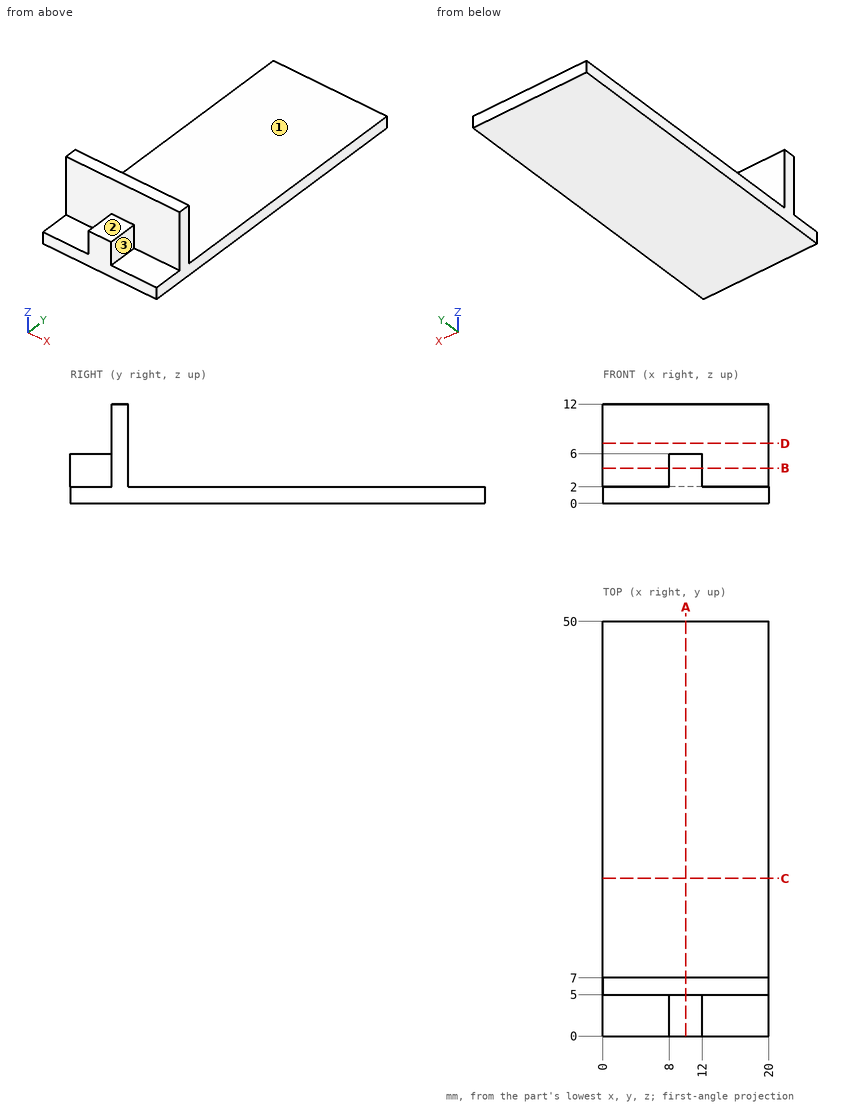
Geometry: see drawing. Coordinates: mm, zero at the bounding-box minimum. A direction names the side the tool comes from. Round coordinates to 2 decimals unless told otherwise and drop trailing zeros. Order: outer loops, then holes, each group sorted by start corner. A loop starts at its lowest first (then second) coordinate and runs counter-clockwise, first axis right, second up. Notation, with made-up numbers: (84, 3) -> (127, 3) arc R18 ccw to (127, 28) -> close; hole circle Ø7 at (86.5, -25.5). An arc over 180 degrees is marked (long way). Answer as CSV lines item,"result".
Item 1: Line query: L1, parallel to Z at x = 1.75, y = 20; L2, parallel to Y at x = 17.5, z = 11. Output: solid intervals per line, ascending.
A:
L1,"0 to 2"
L2,"5 to 7"
Item 2: Section B-B, the plane z = 4.25. Return loops of the section in (x, y), plus the area to 3 significant figures.
A:
outline,"(0, 5) -> (8, 5) -> (8, 0) -> (12, 0) -> (12, 5) -> (20, 5) -> (20, 7) -> (0, 7) -> close"
area,"60.0 mm²"
Item 3: Section A-A, the plane x = 10. Return loops of the section in (y, z).
A:
outline,"(0, 0) -> (50, 0) -> (50, 2) -> (7, 2) -> (7, 12) -> (5, 12) -> (5, 6) -> (0, 6) -> close"
Item 4: Pin query (flat end, axial travel): pin 1 Ø1.5 at (x, y) = (9.5, 13.5) entering from -Z; pin 2 Ø2 at (x, y) = (11, 1.5) entering from +Z; pin 3 Ø6 at (x, y) = (13.5, 24) entering from +Z. Return the tip coordinate at first contact, or that it passes through.
A:
pin 1,"z = 0"
pin 2,"z = 6"
pin 3,"z = 2"
Item 5: Section D-D, the plane z = 7.25. Return loops of the section in (x, y), plus the area to 3 significant figures.
A:
outline,"(0, 5) -> (20, 5) -> (20, 7) -> (0, 7) -> close"
area,"40.0 mm²"
Item 6: Section C-C, the plane y = 19. Return loops of the section in (x, z).
A:
outline,"(0, 0) -> (20, 0) -> (20, 2) -> (0, 2) -> close"
Item 7: Reachability of the marked faces 1, 2 and 3 from +Z, -Z, +X, -X, +Y, -Y: full face, straight path, thin tool, end or side. Return the list, or none.
A:
face 1,"+Z, +X, -X, +Y"
face 2,"+Z, +X, -X, -Y"
face 3,"+Z, +X, -Y"
